Check sheet for the modelled part. Datum: model origin and axes. Units: mm. A direction names the side the tool comes from. Coordinates: 2 decimals unless noted, no trailing zeros. Write each loop counter-clockwise with the first axis right and the second up, starting at its lowest first coordinate (ties: lowest second). Pieces come first, ordered by that corner, then holes. Notation, with made-up numbers: M 52.5,-27.75 L 75.5,-27.75 A19 cw 75.5,5.25 Z; hole C 44,1 d10. An arc over 180 degrees is marked long. Answer as CSV lines item,"result".
from build123d import *

# Parameters (mm, degrees)
BOSS_EXTRUDE1_DEPTH = 4


with BuildPart() as part:
    # Sketch2 → Boss-Extrude1 (new body)
    with BuildSketch(Plane.XY):
        with BuildLine():
            Line((-59, 31), (-59, -31))
            ThreePointArc((-59, -31), (-58.996474756, -31.265504145), (-58.98590151, -31.530821096))
            ThreePointArc((-58.98590151, -31.530821096), (-59.328144398, -33.323028098), (-60.464454078, -34.750591212))
            ThreePointArc((-60.464454078, -34.750591212), (-60.995689014, -42.995689014), (-52.750591212, -42.464454078))
            ThreePointArc((-52.750591212, -42.464454078), (-51.323028098, -41.328144398), (-49.530821096, -40.98590151))
            ThreePointArc((-49.530821096, -40.98590151), (-49.265504145, -40.996474756), (-49, -41))
            Line((-49, -41), (49, -41))
            ThreePointArc((49, -41), (49.265504145, -40.996474756), (49.530821096, -40.98590151))
            ThreePointArc((49.530821096, -40.98590151), (51.323028098, -41.328144398), (52.750591212, -42.464454078))
            ThreePointArc((52.750591212, -42.464454078), (60.995689014, -42.995689014), (60.464454078, -34.750591212))
            ThreePointArc((60.464454078, -34.750591212), (59.328144398, -33.323028098), (58.98590151, -31.530821096))
            ThreePointArc((58.98590151, -31.530821096), (58.996474756, -31.265504145), (59, -31))
            Line((59, -31), (59, 31))
            ThreePointArc((59, 31), (58.996474756, 31.265504145), (58.98590151, 31.530821096))
            ThreePointArc((58.98590151, 31.530821096), (59.328144398, 33.323028098), (60.464454078, 34.750591212))
            ThreePointArc((60.464454078, 34.750591212), (60.995689014, 42.995689014), (52.750591212, 42.464454078))
            ThreePointArc((52.750591212, 42.464454078), (51.323028098, 41.328144398), (49.530821096, 40.98590151))
            ThreePointArc((49.530821096, 40.98590151), (49.265504145, 40.996474756), (49, 41))
            Line((49, 41), (-49, 41))
            ThreePointArc((-49, 41), (-49.265504145, 40.996474756), (-49.530821096, 40.98590151))
            ThreePointArc((-49.530821096, 40.98590151), (-51.323028098, 41.328144398), (-52.750591212, 42.464454078))
            ThreePointArc((-52.750591212, 42.464454078), (-60.995689014, 42.995689014), (-60.464454078, 34.750591212))
            ThreePointArc((-60.464454078, 34.750591212), (-59.328144398, 33.323028098), (-58.98590151, 31.530821096))
            ThreePointArc((-58.98590151, 31.530821096), (-58.996474756, 31.265504145), (-59, 31))
        make_face()
    extrude(amount=BOSS_EXTRUDE1_DEPTH)


solid = part.part
1) Tool access check on faces 5 (the face through (60.9, -43.09, 1.97)), 6 (the face through (59.317, 33.3, 1.972)), 7 (the face through (51.35, 41.34, 1.97)), 8 (the face through (-59.317, -33.3, 1.972)). Record the directions out of +Z, -Z, +X, -X, +Y, -Y that give a thin tool (end or side, any length) a straight path to the whole face; none if there is none.
Answer key:
face 5,"+Z, -Z"
face 6,"+Z, -Z, +X"
face 7,"+Z, -Z, +Y"
face 8,"+Z, -Z, -X"
2) Depth check by flat-ended pin: P1, Ø2, axis at y = -0.5, z = 1.5, coming from the +X side; P2, Ø1.5, axis at x = 25, z = 3, coming from the -Y side; P3, Ø1, axis at y = -22, z = 3, coming from the -X side. Enter the tip coordinate at first touch or a pass-through.
Answer key:
P1,"stops at x = 59"
P2,"stops at y = -41"
P3,"stops at x = -59"
3) Section check B-B, the plane x = -27. Record the boundary of the cut face in (y, z).
Answer key:
outline,"M -41,0 L 41,0 L 41,4 L -41,4 Z"
4) Section check A-A, the plane z = 2.95. Record the boundary of the cut face in (x, y), plus the area to 3 significant figures.
Answer key:
outline,"M -60.46,-34.75 A5.5 ccw long -52.75,-42.46 A3.81 cw -49.53,-40.99 A10 ccw -49,-41 L 49,-41 A10 ccw 49.53,-40.99 A3.81 cw 52.75,-42.46 A5.5 ccw long 60.46,-34.75 A3.81 cw 58.99,-31.53 A10 ccw 59,-31 L 59,31 A10 ccw 58.99,31.53 A3.81 cw 60.46,34.75 A5.5 ccw long 52.75,42.46 A3.81 cw 49.53,40.99 A10 ccw 49,41 L -49,41 A10 ccw -49.53,40.99 A3.81 cw -52.75,42.46 A5.5 ccw long -60.46,34.75 A3.81 cw -58.99,31.53 A10 ccw -59,31 L -59,-31 A10 ccw -58.99,-31.53 A3.81 cw Z"
area,"9,870 mm2"
5) Mould release check, pull along X, two halves, no side actions. Record for faces 1 (the face through (-1, 1, 0)), 2 (the face through (-51.35, -41.34, 1.97)), 3 (the face through (-1, -41, 2)), 4 (the face through (-59.34, 33.35, 1.97)): pulls with the +X half, pulls with the -X half, needs draft (parallel to the pull), parting line crosses it, or undercut.
Answer key:
face 1,"needs draft"
face 2,"undercut"
face 3,"undercut"
face 4,"pulls with the -X half"
6) Section check C-C, the plane y = 15. Record the boundary of the cut face in (x, z), plus the area to 3 significant figures.
Answer key:
outline,"M -59,0 L 59,0 L 59,4 L -59,4 Z"
area,"472 mm2"
7) Thickness scan on line 1 along X through (y, z) = (25.5, 2.9); line 2 along Y through (x, z) = (-8.5, 2.05); line 3 along Y through (x, z) = (53, 3.5). Record the ranges inside material, lowest first.
Answer key:
line 1,"x = -59 to 59"
line 2,"y = -41 to 41"
line 3,"y = -42.77 to 42.77"
